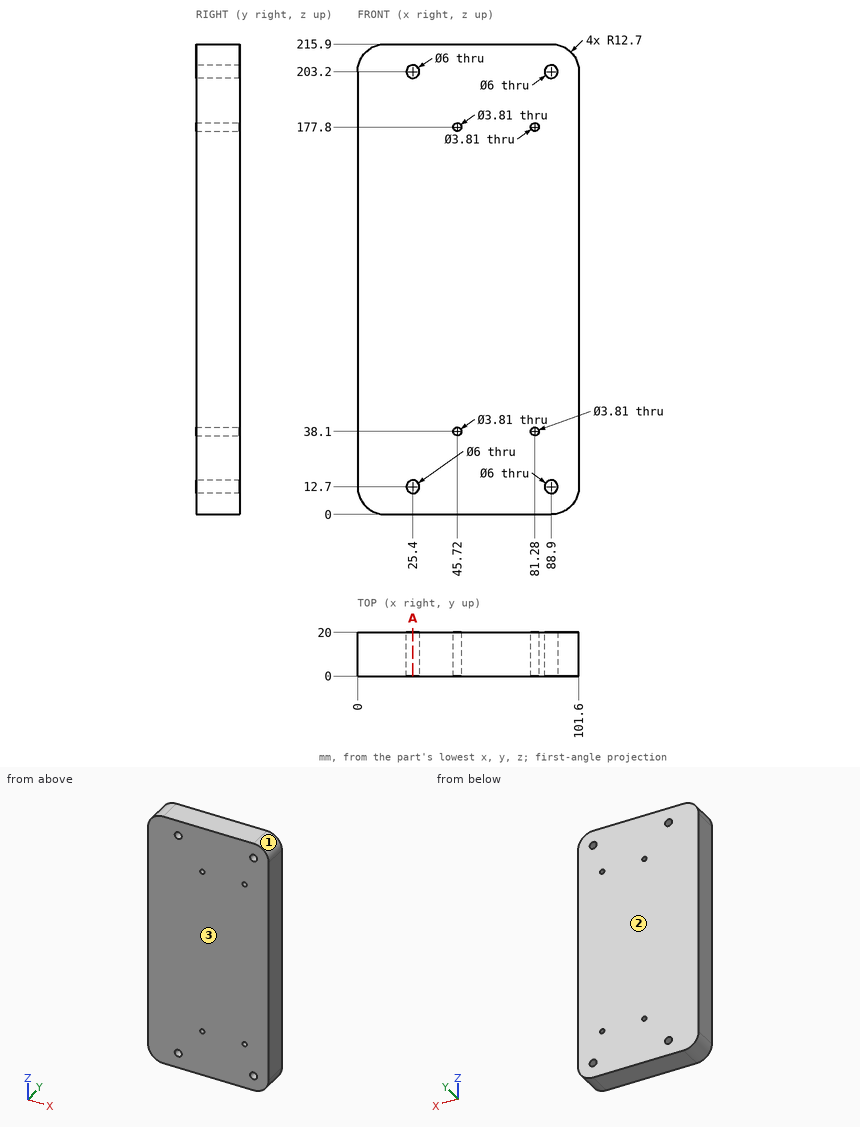
Design review of the part shown in the three views and the two pictorial views. Dimensions are in mm from the part's minimum x, y and z. Round coordinates to 2 decimals unless told otherwise and drop trailing zeros. Write each loop counter-clockwise with the first axis right and the second up, starting at its lowest first coordinate (ties: lowest second). Pieces come first, ordered by that corner, then holes. Notation, with made-up numbers: (73.25, 41) -> (116.25, 41) arc R14 ccw to (116.25, 48) -> close; hole circle Ø9 at (11, -32.75). An arc over 180 degrees is marked (long way). One line per question, with ' | ' between items. Start each with the question number.
1) For pin 1 Ø2.5 at (x, z) = (45.72, 177.8) entering from -Y, flat-tipped, find the tip position at first contact; note if it passes through.
2) Wall thickness on line 1 along X through (y, z) = (11.25, 38.1) (3 decimals); line 2 along Z through (x, y) = (81.28, 14.75) (3 decimals); line 3 along Z through (x, y) = (25.4, 14): over which ranges is each line inside the solid? List them lowest first.
3) Mouldability with a two-part tool opening along Y and no side actions: class the marked faces 1, 2 and 3 as +Y half, -Y half, draft (parallel to the pull), parting line (faces both ways), or undercut.
4) Add section A-A (x = 25.4). Write out the cut boundary in (y, z).
Reported:
1) pin 1: passes through
2) line 1: x = 0 to 43.815, 47.625 to 79.375, 83.185 to 101.6 | line 2: z = 0 to 36.195, 40.005 to 175.895, 179.705 to 215.9 | line 3: z = 0 to 9.7, 15.7 to 200.2, 206.2 to 215.9
3) face 1: draft | face 2: +Y half | face 3: -Y half
4) outline: (0, 0) -> (20, 0) -> (20, 9.7) -> (0, 9.7) -> close; (0, 15.7) -> (20, 15.7) -> (20, 200.2) -> (0, 200.2) -> close; (0, 206.2) -> (20, 206.2) -> (20, 215.9) -> (0, 215.9) -> close
